Can you work these out from the model? Positions are in its coordinate system, mm. A direction names the side the tool comes from. Give positions to 0.01 mm unless a question says otherwise; leave off trailing zeros. Loops run counter-clockwise (first coordinate to the right, second up) from the corner with the lowest first, then second, coordinate; pieces in that order, holes last. Notation, with made-up numbers: (-27, 79) - (19, 79) arc R26 ccw to (19, 105) - close; hole circle Ø1 at (-1, 37). An arc over 180 degrees is marked (long way). Answer as a JSON object with one key per item and string values. Group by question number.
Item 1: Please list where these lines run through material, in increasing order: L1, parallel to X at y = -2, z = -9.5; L2, parallel to Z at x = -2.5, y = 7.5; L3, parallel to X at y = -1.25, z = -10.
Item 2: Will these pins go through, and if not, where does the flat tip stop? pin 1 (10 mm diameter, centred on x = 18, z = 6, fed in from +Y); pin 2 (4 mm diameter, centred on x = 17, y = -9, fed in from -Z); pin 3 (3.5 mm diameter, centred on y = 6.364, z = -6.364, fed in from +X); pin 4 (6 mm diameter, centred on x = -10, z = -10, fed in from +Y).
Item 3: Suppose I cut it at A-A on x = 19.5. Write out the boundary of the cut face in (y, z).
Item 4: Thinking about a two-plate mould opening in Z: for faces 1 (the flat face through (24, -2.1, -4.3)), 2 (the cylindrical face through (-6.493, 1.947, -2.539)), 3 (the cylindrical face through (-3.042, -4.392, -4.851)), which applies, pulls with the +Z half, pulls with the -Z half, needs draft (parallel to the pull), parting line crosses it, or undercut?
Item 5: Which directions (+Z, -Z, +X, -X, +Y, -Y) give clear straight access to the entire face, cutting with the end or side of a thin tool? Please do faces 4 (the flat face through (26, 0, 0)), 5 (the cylindrical face through (24.986, 4.344, 0.965)), 6 (the flat face through (0, -6, 6)).
Autodesk Inventor part; units mm, degrees
ref_plane "YZ Plane" through (0, 0, 0) normal (1, 0, 0) x (0, 1, 0)
ref_plane "XZ Plane" through (0, 0, 0) normal (0, 1, 0) x (-1, 0, 0)
ref_plane "XY Plane" through (0, 0, 0) normal (0, 0, 1) x (1, 0, 0)
sketch "Эскиз1" plane through (0, 0, 0) normal (1, 0, 0) x (0, 1, 0)
  circle A0 centre (0, 0) radius 14
  dimension "d0" = 28
extrude "Выдавливание1" add sketch "Эскиз1" along normal blind 18
sketch "Эскиз2" plane through (18, 0, 0) normal (1, 0, 0) x (0, 0, -1)
  circle A0 centre (0, 0) radius 14
  dimension "d3" = 28
extrude "Выдавливание2" add sketch "Эскиз2" along normal blind 6
chamfer "Фаска1" distance 4 angle 45 1 edges at (24, 0, 14)
sketch "Эскиз3" plane through (24, 0, 0) normal (1, 0, 0) x (0, 0, -1)
  circle A0 centre (0, 0) radius 4.45
  dimension "d9" = 8.9
extrude "Выдавливание3" add sketch "Эскиз3" along normal blind 2
sketch "Эскиз4" plane through (0, 0, 0) normal (-1, 0, 0) x (0, 0, 1)
  circle A0 centre (0, 0) radius 14
  dimension "d12" = 28
extrude "Выдавливание4" add sketch "Эскиз4" along normal blind 6
chamfer "Фаска2" distance 3 angle 45 1 edges at (-6, 0, -14)
sketch "Эскиз5" plane through (-6, 0, 0) normal (-1, 0, 0) x (0, 0, 1)
  circle A0 centre (0, 0) radius 3.2
  dimension "d18" = 6.4
extrude "Выдавливание5" add sketch "Эскиз5" along normal blind 1
sketch "Эскиз6" plane through (-7, 0, 0) normal (-1, 0, 0) x (0, 0, 1)
  circle A0 centre (0, 0) radius 2
  dimension "d21" = 4
extrude "Выдавливание6" add sketch "Эскиз6" along normal blind 11
sketch "Эскиз7" plane through (-6, 0, 0) normal (-1, 0, 0) x (0, 0, 1)
  circle A0 centre (5.6569, 5.6569) radius 1.5
  line L0 (0, 0) -> (14, 0) construction
  circle A1 centre (0, 0) radius 14 construction
  line L1 (0, 0) -> (0, 14) construction
  line L2 (-4.7873, -4.7873) -> (5.6569, 5.6569) construction
  circle A2 centre (0, 0) radius 2 construction
  line L3 (-6.364, 6.364) -> (6.364, -6.364) construction
  circle A3 centre (-6.364, 6.364) radius 1.5
  circle A4 centre (6.364, -6.364) radius 1.5
  circle A5 centre (-5.6569, -5.6569) radius 1.5
  circle A6 centre (0, 0) radius 14 construction
  dimension "d24" = 3
  dimension "d29" = 45
  dimension "d30" = 3
  dimension "d31" = 16
  dimension "d32" = 18
extrude "Выдавливание7" cut sketch "Эскиз7" against normal blind 6
properties part number "motor_sketch"
Worked out:
{
 "1": {"L1": "x = -6 to 24", "L2": "z = -11.82 to -7.34, -5.38 to 11.82", "L3": "x = -6 to 23.92"},
 "2": {"pin 1": "stops at y = 13.96", "pin 2": "stops at z = -12.12", "pin 3": "stops at x = 24", "pin 4": "passes through"},
 "3": {"outline": "circle Ø28 at (0, 0)"},
 "4": {"face 1": "needs draft", "face 2": "parting line crosses it", "face 3": "undercut"},
 "5": {"face 4": "+Z, -Z, +X, +Y, -Y", "face 5": "+X", "face 6": "-X"}
}
